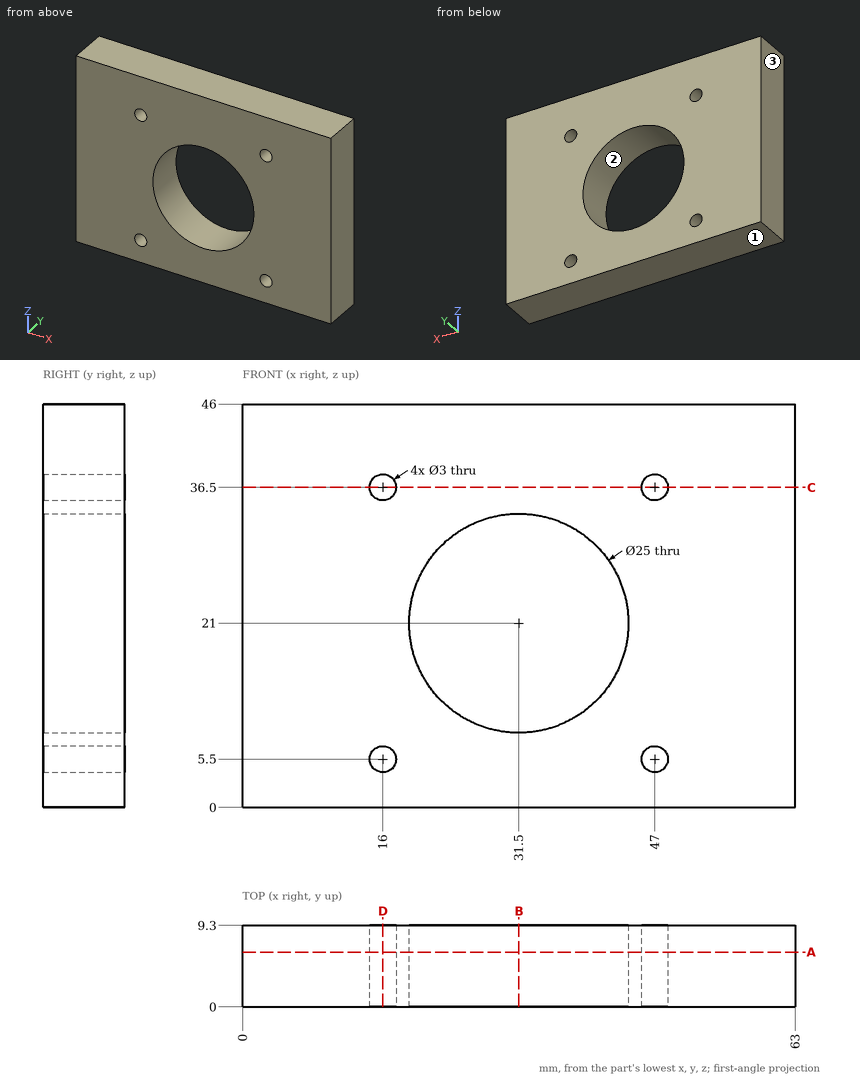
Check sheet for the drawn part. Datum: minimum x, y, z corner. Units: mm. Round coordinates to 2 decimals unless told otherwise and drop trailing zeros. Order: outer loops, then holes, each group sorted by start corner. A loop starts at its lowest first (then second) coordinate and runs counter-clockwise, first axis right, second up. Notation, with made-up numbers: (57.5, 55) - (112.5, 55) arc R25 cw to (112.5, 79) - close; hole circle Ø1 at (30, -20.5). An arc over 180 degrees is marked (long way). Use a Markdown table: item, result. Add a question column.
(1) Sectioned sample at A-A, the plane y = 6.25. Enter the section's corners in (x, z), and give its area (3 significant figures).
(2) Sectioned sample at B-B, the plane x = 31.5. Enter the section's corners in (y, z), and give its area (3 significant figures).
(3) Material ranges on line 1 along X through (y, z) = (4.75, 36.5); line 2 along Z through (x, y) = (16, 5.75); line 3 along Z through (x, y) = (31.5, 7.25), recorded low to high. Write a range as [from, to].
(4) Sectioned sample at C-C, the plane z = 36.5. Enter the section's corners in (x, y).
(5) Depth check by flat-ended pin: pin 1 (1.5 mm diameter, centred on x = 51.5, y = 8, fed in from -Z); pin 2 (2.5 mm diameter, centred on x = 16, z = 36.5, fed in from +Y). Enter the tip coordinate at first touch or a pass-through.
(6) Sectioned sample at D-D, the plane x = 16. Enter the section's corners in (y, z), and give its area (3 significant figures).
(7) Release check for a two-part mould opening along Z. For the marked faces 1, 2 and 3 record: pulls with the +Z half, pulls with the -Z half, needs draft (parallel to the pull), parting line crosses it, or undercut.
Answers below:
| question | item | result |
|---|---|---|
| 1 | outline | (0, 0) - (63, 0) - (63, 46) - (0, 46) - close; hole circle Ø3 at (16, 5.5); hole circle Ø3 at (16, 36.5); hole circle Ø25 at (31.5, 21); hole circle Ø3 at (47, 5.5); hole circle Ø3 at (47, 36.5) |
| 1 | area | 2,380 mm² |
| 2 | outline | (0, 0) - (9.3, 0) - (9.3, 8.5) - (0, 8.5) - close; (0, 33.5) - (9.3, 33.5) - (9.3, 46) - (0, 46) - close |
| 2 | area | 195 mm² |
| 3 | line 1 | [0, 14.5], [17.5, 45.5], [48.5, 63] |
| 3 | line 2 | [0, 4], [7, 35], [38, 46] |
| 3 | line 3 | [0, 8.5], [33.5, 46] |
| 4 | outline | (0, 0) - (14.5, 0) - (14.5, 9.3) - (0, 9.3) - close; (17.5, 0) - (45.5, 0) - (45.5, 9.3) - (17.5, 9.3) - close; (48.5, 0) - (63, 0) - (63, 9.3) - (48.5, 9.3) - close |
| 5 | pin 1 | z = 0 |
| 5 | pin 2 | through |
| 6 | outline | (0, 0) - (9.3, 0) - (9.3, 4) - (0, 4) - close; (0, 7) - (9.3, 7) - (9.3, 35) - (0, 35) - close; (0, 38) - (9.3, 38) - (9.3, 46) - (0, 46) - close |
| 6 | area | 372 mm² |
| 7 | face 1 | pulls with the -Z half |
| 7 | face 2 | undercut |
| 7 | face 3 | needs draft |
